Source: CAD feature listing. Evaluate the final solid. Frame: model axes, mm. A direction names the side the tool comes from. Round coordinates to 2 decimals unless told otherwise and drop trailing zeros. Write each loop counter-clockwise with the first axis right and the second up, starting at its lowest first coordinate (ties: lowest second). Pieces come first, ordered by that corner, then holes. Notation, with made-up numbers: (-32.75, 57.5) -> (-2.75, 57.5) arc R19 cw to (-2.75, 73.5) -> close; hole circle Ø1 at (41, -4.75). An arc over 180 degrees is marked (long way). Put each result on its own line as item: value.
```python
from build123d import *

# Parameters (mm, degrees)
BASE_FLANGE1_DEPTH   = 2
EDGE_FLANGE1_START   = -23
EDGE_FLANGE1_DEPTH   = 46
EDGE_FLANGE1_START_2 = -23.714787909
EDGE_FLANGE1_2_DEPTH = 0.714787909
EDGE_FLANGE1_START_3 = 23
EDGE_FLANGE1_3_DEPTH = 0.714787909
EDGE_FLANGE1_4_DEPTH = 46
CUT_EXTRUDE1_DEPTH   = 10
FILLET1_R            = 4
FILLET2_R            = 6
SKETCH9_R            = 3
CUT_EXTRUDE2_DEPTH   = 10
SKETCH10_R           = 3
BOSS_EXTRUDE1_DEPTH  = 2


# Read off the part's stored shape, not the designer's step: Edge-Flange1
# Sheet-metal steps are written as plain solids
with BuildPart() as part:
    # Sketch1 → Base-Flange1 (new body)
    with BuildSketch(Plane(origin=(0, 0, 0), x_dir=(1, 0, 0), z_dir=(0, 1, 0))):
        with BuildLine():
            Line((-16.949747468, 6.379735664), (-9, -1.570011804))
            Line((-9, -1.570011804), (9, -1.570011804))
            Line((9, -1.570011804), (16.949747468, 6.379735664))
            ThreePointArc((16.949747468, 6.379735664), (19.22071091, 7.897144924), (21.899494937, 8.429988196))
            Line((21.899494937, 8.429988196), (24, 8.429988196))
            ThreePointArc((24, 8.429988196), (27.535533906, 6.965522102), (29, 3.429988196))
            Line((29, 3.429988196), (29, -1.361639596))
            ThreePointArc((29, -1.361639596), (28.339066725, -3.564054954), (26.574683296, -5.038645514))
            Line((26.574683296, -5.038645514), (23, -6.569508994))
            Line((23, -6.569508994), (23, -10))
            Line((23, -10), (-23, -10))
            Line((-23, -10), (-23, -6.569508994))
            Line((-23, -6.569508994), (-26.574683296, -5.038645514))
            ThreePointArc((-26.574683296, -5.038645514), (-28.339066725, -3.564054954), (-29, -1.361639596))
            Line((-29, -1.361639596), (-29, 3.429988196))
            ThreePointArc((-29, 3.429988196), (-27.535533906, 6.965522102), (-24, 8.429988196))
            Line((-24, 8.429988196), (-21.899494937, 8.429988196))
            ThreePointArc((-21.899494937, 8.429988196), (-19.22071091, 7.897144924), (-16.949747468, 6.379735664))
        make_face()
    extrude(amount=-BASE_FLANGE1_DEPTH)

    # Edge-Flange1 outline → Edge-Flange1 (cut)
    with BuildSketch(Plane.YZ.offset(EDGE_FLANGE1_START)):
        with BuildLine():
            ThreePointArc((-2, 9.899002398), (-0.556604688, 8.917667209), (0, 7.2634))
            Line((0, 7.2634), (0, 10))
            Line((0, 10), (-2, 10))
            Line((-2, 10), (-2, 9.899002398))
        make_face()
    extrude(amount=EDGE_FLANGE1_DEPTH, mode=Mode.SUBTRACT)

    # Edge-Flange1 2 outline → Edge-Flange1 2 (cut)
    with BuildSketch(Plane.YZ.offset(EDGE_FLANGE1_START_2)):
        with BuildLine():
            Line((-2, 6.2634), (0, 6.2634))
            Line((0, 6.2634), (0, 7.2634))
            ThreePointArc((0, 7.2634), (-0.556604688, 8.917667209), (-2, 9.899002398))
            Line((-2, 9.899002398), (-2, 6.2634))
        make_face()
    extrude(amount=EDGE_FLANGE1_2_DEPTH, mode=Mode.SUBTRACT)

    # Edge-Flange1 3 outline → Edge-Flange1 3 (cut)
    with BuildSketch(Plane.YZ.offset(EDGE_FLANGE1_START_3)):
        with BuildLine():
            Line((-2, 6.2634), (0, 6.2634))
            Line((0, 6.2634), (0, 7.2634))
            ThreePointArc((0, 7.2634), (-0.556604688, 8.917667209), (-2, 9.899002398))
            Line((-2, 9.899002398), (-2, 6.2634))
        make_face()
    extrude(amount=EDGE_FLANGE1_3_DEPTH, mode=Mode.SUBTRACT)

    # Edge-Flange1 4 outline → Edge-Flange1 4 (add)
    with BuildSketch(Plane.YZ.offset(EDGE_FLANGE1_START)):
        with BuildLine():
            ThreePointArc((-2.7366, 8), (-2.215745145, 7.784254855), (-2, 7.2634))
            Line((-2, 7.2634), (-2, 9.899002398))
            ThreePointArc((-2, 9.899002398), (-2.364854094, 9.974633029), (-2.7366, 10))
            Line((-2.7366, 10), (-15, 10))
            Line((-15, 10), (-15, 8))
            Line((-15, 8), (-2.7366, 8))
        make_face()
    extrude(amount=EDGE_FLANGE1_4_DEPTH)

    # Sketch8 → Cut-Extrude1 (cut)
    with BuildSketch(Plane.XY.offset(10)):
        Polygon((-16, -10), (-23, -3), (-23, -15), (-5, -15), (-10, -10), align=None)
        Polygon((10, -10), (5, -15), (23, -15), (23, -3), (16, -10), align=None)
    extrude(amount=-CUT_EXTRUDE1_DEPTH, mode=Mode.SUBTRACT)

    # Fillet1
    fillet1_edges = [part.edges().sort_by_distance(p)[0] for p in [
        (-23, -3, 9),
        (-16, -10, 9),
        (-10, -10, 9),
        (10, -10, 9),
        (16, -10, 9),
        (23, -3, 9),
    ]]
    fillet(fillet1_edges, radius=FILLET1_R)

    # Fillet2
    fillet2_edges = [part.edges().sort_by_distance(p)[0] for p in [
        (-5, -15, 9),
        (5, -15, 9),
        (9, -1, 1.570011804),
        (-9, -1, 1.570011804),
    ]]
    fillet(fillet2_edges, radius=FILLET2_R)

    # Sketch9 → Cut-Extrude2 (cut)
    with BuildSketch(Plane.XY.offset(10)):
        with Locations((0, -9)):
            Circle(SKETCH9_R)
    extrude(amount=-CUT_EXTRUDE2_DEPTH, mode=Mode.SUBTRACT)

    # Sketch10 → Boss-Extrude1 (add)
    with BuildSketch(Plane(origin=(0, 0, 8), x_dir=(-1, 0, 0), z_dir=(0, 0, -1))):
        Polygon((5.42709253, -9), (2.713546265, -4.3), (-2.713546265, -4.3), (-5.42709253, -9), (-2.713546265, -13.7), (2.713546265, -13.7), align=None)
        with Locations(Location((0, -9, 0), (0, 0, 180))):
            Circle(SKETCH10_R, mode=Mode.SUBTRACT)
    extrude(amount=BOSS_EXTRUDE1_DEPTH)


solid = part.part
```
Q1. Pin query (flat end, axial travel): pin 1 (0.6 mm diameter, centred on x = -23, y = -1, fed in from +Z); pin 2 (1.6 mm diameter, centred on x = 0.5, z = 6.5, fed in from -Y); pin 3 (1 mm diameter, centred on x = 13.5, z = 9, fed in from -Y); pin 4 (8 mm diameter, centred on x = 4.5, z = -3.5, fed in from -Y). Return the tip coordinate at first contact, or that it passes through.
Ans:
pin 1: stops at z = 9.59
pin 2: stops at y = -13.7
pin 3: stops at y = -10
pin 4: passes through
Q2. Draft query along X for faces 5 (the flat face through (-4.051, -11.383, 7.014)), 6 (the flat face through (4.1, -11.3, 7)), 7 (the cylindrical face through (8.78, -1.014, 1.126)). Return one class per face: +X half, -X half, draft (parallel to the pull), parting line (faces both ways), or undercut.
Ans:
face 5: -X half
face 6: +X half
face 7: undercut
Q3. Cut plane A-A on x = 0. Output: boundary loops of the cut face in (y, z), and give its area (3 significant figures).
Ans:
outline: (-15, 8) -> (-13.7, 8) -> (-13.7, 6) -> (-12, 6) -> (-12, 10) -> (-15, 10) -> close; (-6, 6) -> (-4.3, 6) -> (-4.3, 8) -> (-2.74, 8) arc R0.74 cw to (-2, 7.26) -> (-2, 1.57) -> (0, 1.57) -> (0, 7.26) arc R2.74 ccw to (-2.74, 10) -> (-6, 10) -> close
area: 36.2 mm^2
Q4. Reachability of faces 1 (the flat face through (13, -10, 9)), 2 (the cylindrical face through (-19.256, -0.986, -7.912)), 3 (the flat face through (0, -4.3, 7)), 4 (the flat face through (0, -13.7, 7)) from +Z, -Z, +X, -X, +Y, -Y: full face, straight path, thin tool, end or side. Return the list, or none.
Ans:
face 1: +Z, -Z, +X, -Y
face 2: -Z, +Y, -Y
face 3: -Z, +X, -X
face 4: -Z, +X, -X, -Y
Q5. Cut plane B-B on z = -4. Output: boundary loops of the cut face in (x, y), and give its area (3 significant figures).
Ans:
outline: (-28.97, -2) -> (-14.57, -2) -> (-14.57, 0) -> (-28.97, 0) -> close; (14.57, -2) -> (28.97, -2) -> (28.97, 0) -> (14.57, 0) -> close
area: 57.6 mm^2
Q6. Material intervals for line 1 (Y direction, x = 0, z = 7); line 2 (X direction, y = -9, z = 7.55); line 3 (Y direction, x = 0, z = 7.7), sorted ascending. Write a range as [from, to].
Ans:
line 1: y = [-13.7, -12], [-6, -4.3], [-2, 0]
line 2: x = [-5.43, -3], [3, 5.43]
line 3: y = [-13.7, -12], [-6, -4.3], [-2.14, -0.04]
Q7. Cut plane C-C on z = 3.75. Output: boundary loops of the cut face in (x, y), and give its area (3 significant figures).
Ans:
outline: (-28.21, -2) -> (28.21, -2) -> (28.21, 0) -> (-28.21, 0) -> close
area: 113 mm^2
